Solid Edge part; units mm, degrees
sketch "Sketch1" plane through (0, 0, 0) normal (0, 0, 1) x (1, 0, 0)
  arc A0 (20.4574, 11) -> (20.4574, -11) centre (11.7971, 0) cw
  line L0 (-20.4574, -11) -> (20.4574, -11)
  arc A1 (-20.4574, 11) -> (-20.4574, -11) centre (-11.7971, 0) ccw
  line L1 (-20.4574, 11) -> (20.4574, 11)
extrude "Ajout_matière_1" add sketch "Sketch1" against normal blind 24
sketch "Sketch2" plane through (0, 0, 0) normal (0, 0, 1) x (-1, 0, 0)
  circle A0 centre (10, 0) radius 8.2
  circle A1 centre (-10, 0) radius 8.2
extrude "Cutout1" cut sketch "Sketch2" against normal through all and the other way up to next
fillet "Congé_1" radius 7 4 edges at (20.4574, -11, -12) (20.4574, 11, -12) (-20.4574, 11, -12) (-20.4574, -11, -12)
sketch "Sketch3" plane through (0, 11, -10) normal (0, 1, 0) x (-1, 0, 0)
  line L0 (-20.4139, 10) -> (20.4139, 10)
  line L1 (20.4139, 10) -> (20.4139, -14)
  line L2 (20.4139, -14) -> (-20.4139, -14)
  line L3 (-20.4139, -14) -> (-20.4139, 10)
extrude "Ajout_matière_3" add sketch "Sketch3" along normal blind 15 and the other way up to next
hole "Perçage_3" at (6, 17.8836, 0) direction (0, 0, -1) diameter 5 end up to next
hole "Hole1" at (-6, 17.8836, 0) direction (0, 0, -1) diameter 5 end up to next
sketch "Sketch4" plane through (0, 26, -10) normal (0, 1, 0) x (-1, 0, 0)
  line L0 (-14.5, 5.5) -> (-14.5, -9.5)
  line L1 (-14.5, -9.5) -> (14.5, -9.5)
  line L2 (14.5, -9.5) -> (14.5, 5.5)
  line L3 (14.5, 5.5) -> (-14.5, 5.5)
  dimension "D1" = 14.5
  dimension "D2" = 14.5
extrude "Enlèvement_matière_3" cut sketch "Sketch4" against normal blind 15
chamfer "Chanfrein_3" distance 1 angle 45 18 edges at (25.7971, 0, 0) (20.782, -10.2048, 0) (0, -11, 0) (-20.782, -10.2048, 0) (-25.7971, 0, 0) (-22.0119, 9.3868, 0) (22.0119, 9.3868, 0) (0, 26, 0) (25.7971, 0, -24) (20.782, -10.2048, -24) (0, -11, -24) (-20.782, -10.2048, -24) (-25.7971, 0, -24) (-22.0119, 9.3868, -24) (22.0119, 9.3868, -24) (0, 26, -24) (-20.4139, 26, -12) (20.4139, 26, -12)
properties material "Plastique ABS, haute performance"
Verification items for the finished model (mm, model axes). A direction names the side the tool comes from. Give positions to 0.01 mm unless a question says otherwise; leave off trailing zeros. Loops run counter-clockwise (first coordinate to the right, second up) from the corner with the lowest first, then second, coordinate; pieces in that order, holes last.
1) Sectioned sample at C-C, the plane y = 0. Enter the section's corners in (x, z).
2) Draft check along X on faces 3 (the flat face through (0, 8, -24)), 4 (the flat face through (14.5, 19, -12)), 5 (the cylindrical face through (20.824, -10.183, -12.154)), 6 (the cylindrical face through (-20.74, -10.227, -12.154)). Enter one of: pulls with the +X half, pulls with the -X half, needs draft (parallel to the pull), parting line crosses it, or undercut.
3) Thickness scan on line 1 along X through (y, z) = (0, -20.25); line 2 along Z through (x, y) = (-1, 20); line 3 along Y through (x, z) = (10, -10). Record the ranges inside material, lowest first.
4) Sectioned sample at D-D, the plane x = 1. Enter the section's corners in (y, z), then the cut area to 3 significant figures.
5) Set-up check for faces 1 (the flat face through (0, -11, -12)), 2 (the flat face through (0, 11, -12)): record each of +Z, -Z, +X, -X, +Y, -Y from which the full face is reachable in a straight line by a thin tool's end or side.
6) Sectioned sample at A-A, the plane x = 10. Enter the section's corners in (y, z), then the cut area to 3 significant figures.
7) Depth check by flat-ended pin: pin 1 Ø4.5 at (x, y) = (6, 17.88) entering from -Z; pin 2 Ø1 at (y, z) = (15, -14.5) entering from -X; pin 3 Ø7.5 at (x, y) = (5, 18) entering from -Z; pin 4 Ø12.5 at (y, z) = (19, -7) entering from +X. Enter the tip coordinate at first touch or a pass-through.
8) Sectioned sample at B-B, the plane z = -20.5. Enter the section's corners in (x, y), then the cut area to 3 significant figures.
Answers:
1. outline: (-25.8, -23) - (-24.8, -24) - (-18.2, -24) - (-18.2, 0) - (-24.8, 0) - (-25.8, -1) - close; (-1.8, -24) - (1.8, -24) - (1.8, 0) - (-1.8, 0) - close; (18.2, -24) - (24.8, -24) - (25.8, -23) - (25.8, -1) - (24.8, 0) - (18.2, 0) - close
2. face 3: needs draft
2. face 4: undercut
2. face 5: pulls with the +X half
2. face 6: pulls with the -X half
3. line 1: x = -25.8 to -18.2, -1.8 to 1.8, 18.2 to 25.8
3. line 2: z = -24 to -19.5, -4.5 to 0
3. line 3: y = -11 to -8.2, 8.2 to 11
4. outline: (-11, -23) - (-10, -24) - (25, -24) - (26, -23) - (26, -19.5) - (11, -19.5) - (11, -4.5) - (26, -4.5) - (26, -1) - (25, 0) - (-10, 0) - (-11, -1) - close
4. area: 661 mm2
5. face 1: +Z, -Z, +X, -X, -Y
5. face 2: +Y
6. outline: (-11, -23) - (-10, -24) - (-8.2, -24) - (-8.2, 0) - (-10, 0) - (-11, -1) - close; (8.2, -24) - (25, -24) - (26, -23) - (26, -19.5) - (11, -19.5) - (11, -4.5) - (26, -4.5) - (26, -1) - (25, 0) - (8.2, 0) - close
6. area: 267 mm2
7. pin 1: passes through
7. pin 2: stops at x = -20.41
7. pin 3: stops at z = -24
7. pin 4: stops at x = 20.41
8. outline: (-23.29, -8) arc R7 ccw to (-17.54, -11) - (17.54, -11) arc R7 ccw to (23.29, -8) arc R14 ccw to (23.29, 8) arc R7 ccw to (20.41, 10.38) - (20.41, 25) - (19.41, 26) - (-19.41, 26) - (-20.41, 25) - (-20.41, 10.38) arc R7 ccw to (-23.29, 8) arc R14 ccw to start; hole circle Ø16.4 at (-10, 0); hole circle Ø5 at (-6, 17.88); hole circle Ø16.4 at (10, 0); hole circle Ø5 at (6, 17.88)
8. area: 1,210 mm2
